Autodesk Inventor part; units mm, degrees
ref_plane "Work Plane1" through (0, 3, 0) normal (0, 1, 0) x (-1, 0, 0)
ref_plane "YZ Plane" through (0, 0, 0) normal (1, 0, 0) x (0, 1, 0)
ref_plane "XY Plane" through (0, 0, 0) normal (0, 0, 1) x (1, 0, 0)
sketch "Sketch1" plane through (0, 0, 0) normal (0, 0, 1) x (1, 0, 0)
  circle A0 centre (0, 0) radius 70
  arc A1 (40.7232, -41.2992) -> (-40.7232, -41.2992) centre (0, 0) ccw
  arc A2 (-4.75, -8.6033) -> (4.75, -8.6033) centre (0, -27) ccw
  circle A3 centre (0, -27) radius 30
  arc A4 (29.0338, -34.5526) -> (40.7232, -41.2992) centre (35.8083, -36.3148) ccw
  arc A5 (-40.7232, -41.2992) -> (-29.0338, -34.5526) centre (-35.8083, -36.3148) ccw
  line L0 (0, -46) -> (0, -3.8) construction
  line L1 (-4.75, -3.8) -> (4.75, -3.8)
  line L2 (-4.75, -3.8) -> (-4.75, -8.6033)
  line L3 (4.75, -3.8) -> (4.75, -8.6033)
  line L4 (-19, 54.7996) -> (19, 54.7996) construction
  line L5 (-32.5, 20.2582) -> (32.5, 20.2582) construction
  line L6 (0, -98) -> (0, 98) construction
  arc A6 (15.5233, 6.0625) -> (20.7447, -5.3284) centre (32.5, 6.9522) ccw
  arc A7 (21.5482, 53.8486) -> (13.3273, 47.9641) centre (19.3191, 48.2781) ccw
  line L7 (13.3273, 47.9641) -> (15.5233, 6.0625)
  arc A8 (-13.3273, 47.9641) -> (-21.5482, 53.8486) centre (-19.3191, 48.2781) ccw
  arc A9 (-20.7447, -5.3284) -> (-15.5233, 6.0625) centre (-32.5, 6.9522) ccw
  line L8 (-13.3273, 47.9641) -> (-15.5233, 6.0625)
  point P0 (0, -3.8)
  point P1 (0, 20.2582)
  dimension "d0" = 70
  dimension "d1" = 58
  dimension "d2" = 19
  dimension "d3" = 30
  dimension "d4" = 27
  dimension "d5" = 42.2
  dimension "d6" = 9.5
  dimension "d7" = 38
  dimension "d8" = 65
  dimension "d13" = 7
  dimension "d14" = 7
  dimension "d15" = 3.8
  dimension "d16" = 17
  dimension "d17" = 6
  dimension "d18" = 3
  dimension "d19" = 6
  dimension "d20" = 17
  dimension "d21" = 3
extrude "Extrusion1" add sketch "Sketch1" along normal mid plane 57.15 contours A3
ref_plane "Work Plane1" through (0, 3, 0) normal (0, 1, 0) x (-1, 0, 0)
sketch "Sketch2" plane through (0, 3, 0) normal (0, 1, 0) x (-1, 0, 0)
  line L0 (30, -28.575) -> (-30, -28.575)
  line L1 (-30, 28.575) -> (30, 28.575)
  line L2 (0, 28.575) -> (0, 9.125)
  line L3 (0, -28.575) -> (0, -3.875)
  point P0 (0, 0)
  dimension "d25" = 19.45
  dimension "d26" = 24.7
  dimension "d27" = 3.875
  dimension "d28" = 9.125
extrude "Extrusion2" add sketch "Sketch1" along normal blind 9.125 and the other way blind 3.875 contours A7 L7 A6 A3 A9 L8 A8 A1
sketch "Sketch3" plane through (0, 3, 0) normal (0, 1, 0) x (-1, 0, 0)
  line L0 (20.7447, -3.875) -> (-20.7447, -3.875)
  line L1 (-20.7447, -3.875) -> (-20.7447, 9.125)
  line L2 (-20.7447, 9.125) -> (20.7447, 9.125)
  line L3 (20.7447, -3.875) -> (20.7447, 9.125)
  line L4 (30, -28.575) -> (-30, -28.575)
  line L5 (-30, 28.575) -> (30, 28.575)
  line L6 (0, 28.575) -> (0, 22.125)
  line L7 (0, -28.575) -> (0, -16.075)
  point P0 (0, 0)
  dimension "d33" = 6.45
  dimension "d34" = 12.5
  dimension "d35" = 22.125
  dimension "d36" = 16.075
extrude "Extrusion3" add sketch "Sketch1" along normal blind 22.125 and the other way blind 16.075 contours A0
chamfer "Chamfer1" distance 3 angle 45 1 edges at (-70, 0, -16.075)
properties part number "Piesa24_DonisanEnya"
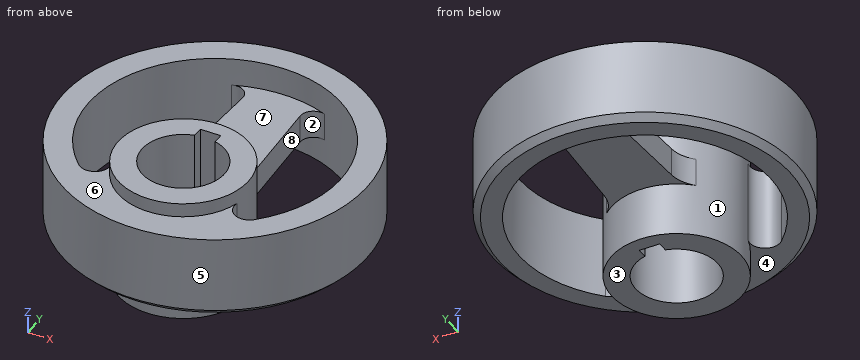
Verification items for the finished model (mm, model axes). Face numbers are marked on the shaded views. A direction names the side the tool comes from. Round coordinates to 2 decimals unless told otherwise and drop trailing zeros. Order: outer loops, then holes, each group sorted by start corner. A loop starts at its lowest first (then second) coordinate and runs counter-clockwise, first axis right, second up. Notation, with made-up numbers: (23.5, 54.25) -> (42.5, 54.25) arc R17 cw to (42.5, 69.25) -> close; hole circle Ø9 at (35, -11.75). An arc over 180 degrees is marked (long way). Put each result on its own line as item: value.
1) Mould release check, pull along Y, two halves, no side actions. Record for the marked faces 5, 6, 7 and 8: +Y half, -Y half, draft (parallel to the pull), parting line (faces both ways), or undercut.
Final values:
face 5: parting line
face 6: draft
face 7: undercut
face 8: undercut
2) Section check A-A (x = 0). Record the cut outline in (y, z) (3 decimals).
Final values:
outline: (-70, -13.075) -> (-67, -16.075) -> (-57, -16.075) -> (-57, -28.575) -> (-46, -28.575) -> (-46, 28.575) -> (-57, 28.575) -> (-57, 22.125) -> (-70, 22.125) -> close; (-3.8, -28.575) -> (3, -28.575) -> (3, -3.875) -> (58, -3.875) -> (58, -16.075) -> (67, -16.075) -> (70, -13.075) -> (70, 22.125) -> (58, 22.125) -> (58, 9.125) -> (3, 9.125) -> (3, 28.575) -> (-3.8, 28.575) -> close
3) Set-up check for the marked faces 1, 2, 3 and 4: record each of +Z, -Z, +X, -X, +Y, -Y from which the full face is reachable in a straight line by a thin tool's end or side.
Final values:
face 1: none
face 2: +Z, -Z
face 3: -Z, +X, -X, +Y, -Y
face 4: -Z
4) Section check D-D (z = -6). Record the cut outline in (x, y), then the cut area to 3 significant figures.
Final values:
outline: circle Ø140 at (0, 0); hole (-40.72, -41.3) arc R7 ccw to (-29.03, -34.55) arc R30 cw (long way) to (29.03, -34.55) arc R7 ccw to (40.72, -41.3) arc R58 ccw (long way) to start; hole (-4.75, -8.6) arc R19 ccw (long way) to (4.75, -8.6) -> (4.75, -3.8) -> (-4.75, -3.8) -> close
area: 6,820 mm^2
5) Section check B-B (z = -20). Record the cut outline in (x, y), then the cut area to 3 significant figures.
Final values:
outline: circle Ø60 at (0, -27); hole (-4.75, -8.6) arc R19 ccw (long way) to (4.75, -8.6) -> (4.75, -3.8) -> (-4.75, -3.8) -> close
area: 1,650 mm^2
6) Section check C-C (y = 0). Record the cut outline in (x, z) (3 decimals), then the cut area to 3 significant figures.
Final values:
outline: (-70, -13.075) -> (-67, -16.075) -> (-58, -16.075) -> (-58, 22.125) -> (-70, 22.125) -> close; (-16.987, -3.875) -> (-13.077, -3.875) -> (-13.077, -28.575) -> (13.077, -28.575) -> (13.077, -3.875) -> (16.987, -3.875) -> (16.987, 9.125) -> (13.077, 9.125) -> (13.077, 28.575) -> (-13.077, 28.575) -> (-13.077, 9.125) -> (-16.987, 9.125) -> close; (58, -16.075) -> (67, -16.075) -> (70, -13.075) -> (70, 22.125) -> (58, 22.125) -> close
area: 2,500 mm^2
7) Depth check by flat-ended pin: pin 1 (12 mm diameter, centred on x = -41.5, z = -18.5, fed in from +Y); pin 2 (21.5 mm diameter, centred on x = 0.5, y = 32, fed in from -Z) (3 decimals); pin 3 (3 mm diameter, centred on y = -10, z = 11, fed in from +X). Enter the tip coordinate at first touch or a pass-through.
Final values:
pin 1: stops at y = 58.19
pin 2: stops at z = -3.875
pin 3: stops at x = 69.48
8) Material ranges on line 1 (Y direction, x = 0, z = 14); line 2 (X direction, y = -17, z = -4.5); line 3 (Y direction, x = 0, z = 8), recorded low to high.
Final values:
line 1: y = -70 to -46, -3.8 to 3, 58 to 70
line 2: x = -67.9 to -55.45, -28.28 to -16.16, 16.16 to 28.28, 55.45 to 67.9
line 3: y = -70 to -46, -3.8 to 70
